The listing builds one solid part. Answer for the finished solid, in the listing's coordinates (mm). Give positions to 0.01 mm unless a question says otherwise; leave off trailing zeros. Write each loop counter-clockwise with the first axis right and the second up, starting at its lowest first coordinate (ties: lowest second). Pieces come first, ordered by that corner, then holes. Notation, with made-up numbers: M 58.5,-19.75 L 102.5,-19.75 A16 ccw 102.5,-1.75 Z; hole C 74,-34.5 d5. An arc over 180 degrees is marked long. Answer as a JSON object with one key per item and string values.
```python
from build123d import *

# Parameters (mm, degrees)
FILLET1_R          = 2.54
SKETCH2_R          = 3.25
CUT_EXTRUDE1_DEPTH = 34.251209752


with BuildPart() as part:
    # Sketch1 → Revolve1 (revolve)
    with BuildSketch(Plane.XY, mode=Mode.PRIVATE) as revolve1_sk:
        Polygon((15.875, 0), (15.875, 6.985), (12.7, 6.985), (12.7, 5.08), (0, 5.08), (0, 0), align=None)
    revolve1 = revolve(revolve1_sk.sketch.rotate(Axis((0, 0, 0), (1, 0, 0)), 90), axis=Axis((0, 0, 0), (1, 0, 0)))

    # Mirror1: Revolve1 across plane
    add(revolve1.mirror(Plane(origin=(0, 0, 0), x_dir=(0, 0, 1), z_dir=(1, 0, 0))))

    # Fillet1
    # the kernel refuses this fillet: 2.54 mm, written as the material it adds along each edge
    with BuildSketch(Plane(origin=(-12.7, 0, 0), x_dir=(0, 0, 1), z_dir=(0, 1, 0))) as fillet1_piece_1:
        with BuildLine():
            CenterArc((7.62, 2.459344425), FILLET1_R, 180, 75.522487814)
            Line((6.985, 0), (6.9723, -0.049186888))
            ThreePointArc((6.9723, -0.049186888), (6.0325, -0.0508), (5.08, -0.0508))
            Line((5.08, -0.0508), (5.0292, 0))
            Line((5.0292, 0), (5.0292, 2.459344425))
            Line((5.0292, 2.459344425), (5.08, 2.459344425))
        make_face()
    revolve(axis=Axis((-12.7, 0, 0), (1, 0, 0)))
    with BuildSketch(Plane(origin=(12.7, 0, 0), x_dir=(0, 0, 1), z_dir=(0, 1, 0))) as fillet1_piece_2:
        with BuildLine():
            CenterArc((7.62, -2.459344425), FILLET1_R, 104.477512186, 75.522487814)
            Line((5.08, -2.459344425), (5.0292, -2.459344425))
            Line((5.0292, -2.459344425), (5.0292, 0))
            Line((5.0292, 0), (5.08, 0.0508))
            ThreePointArc((5.08, 0.0508), (6.0325, 0.0508), (6.9723, 0.049186888))
            Line((6.9723, 0.049186888), (6.985, 0))
        make_face()
    revolve(axis=Axis((12.7, 0, 0), (1, 0, 0)))

    # Sketch2 → Cut-Extrude1 (cut, through all)
    with BuildSketch(Plane(origin=(15.875, 0, 0), x_dir=(0, 0, -1), z_dir=(1, 0, 0))):
        Circle(SKETCH2_R)
    extrude(amount=-CUT_EXTRUDE1_DEPTH, mode=Mode.SUBTRACT)


solid = part.part
```
1. A cutting plane is placed at A-A, the plane y = 0. Give the vertices of the cut face in (x, z) (3 decimals), plus the area to 3 significant figures.
Verdict:
{"outline": "M -15.875,-6.985 L -12.7,-6.985 A2.54 cw -10.241,-5.08 L 10.241,-5.08 A2.54 cw 12.7,-6.985 L 15.875,-6.985 L 15.875,-3.25 L -15.875,-3.25 Z; M -15.875,3.25 L 15.875,3.25 L 15.875,6.985 L 12.7,6.985 A2.54 cw 10.241,5.08 L -10.241,5.08 A2.54 cw -12.7,6.985 L -15.875,6.985 Z", "area": "145 mm2"}
2. The mould has two halves that part along Z. Classify faces 1 (the cylindrical face through (0.222, -1.978, 2.579)), 2 (the cylindrical face through (0.143, -5.037, -0.661)), 3 (the flat face through (15.875, -2, -3)): released by +Z, released by -Z, zero draft, split by the parting line, or undercut.
Verdict:
{"face 1": "undercut", "face 2": "split by the parting line", "face 3": "zero draft"}
3. A cutting plane is placed at C-C, the plane x = -9. Give the vertices of the cut face in (y, z), plus the area to 3 significant figures.
Verdict:
{"outline": "C 0,0 d10.16; hole C 0,0 d6.5", "area": "47.9 mm2"}
4. Flat-ended cylindrical pins translate along their axes: pin 1 (1 mm diameter, centred on x = -4, z = 0, fed in from +Y); pin 2 (8 mm diameter, centred on x = 8.5, z = 1.5, fed in from +Y); pin 3 (2 mm diameter, centred on x = -7.5, z = 5.5, fed in from -Y). Find the tip coordinate at first contact, or state that the pin passes through.
Verdict:
{"pin 1": "stops at y = 5.08", "pin 2": "stops at y = 6.33", "pin 3": "stops at y = -2.36"}
5. A cutting plane is placed at D-D, the plane x = -13. Give the vertices of the cut face in (y, z) (3 decimals).
Verdict:
{"outline": "C 0,0 d13.97; hole C 0,0 d6.5"}
6. Consider line 1 along Y through (x, z) = (-4, 0); line 2 along X through (y, z) = (0.25, 5.5) (3 decimals); line 3 along X through (y, z) = (0.75, 5.5) (3 decimals). Determine where each line is inside the solid, lowest interval first.
Verdict:
{"line 1": "y = -5.08 to -3.25, 3.25 to 5.08", "line 2": "x = -15.875 to -11.648, 11.648 to 15.875", "line 3": "x = -15.875 to -11.714, 11.714 to 15.875"}
